For this review, take the finished solid that the model builds, in its own axes (mm). Round coordinates to 2 decimals unless told otherwise and drop trailing zeros. Order: outer loops, then holes, each group sorted by start corner. A loop starts at its lowest first (then second) coordinate and runs counter-clockwise, first axis right, second up. Notation, with made-up numbers: M 54.25,31.5 L 106.25,31.5 A8 ccw 106.25,41.5 Z; hole C 15,-26 d1. An arc over 180 degrees is marked long. Answer as a JSON object with one key per item and string values.
from build123d import *

# Parameters (mm, degrees)
F1_DEPTH = 250


# Not quite as in the source:
# - a fillet or chamfer that OpenCascade refuses, or shapes differently, is made with other operations: its cross-section is extruded or revolved along the edge and cut away or added


with BuildPart() as f1:
    # F0 (on Front) → F1 (new body)
    with BuildSketch(Plane.XZ):
        with BuildLine():
            ThreePointArc((14.3910080635, 0), (-13.3075418668, 5.4781787619), (10.2202866776, -10.1314783379))
            ThreePointArc((10.2202866776, -10.1314783379), (13.3075418668, -5.4781787619), (14.3910080635, 0))
        make_face()
        with BuildLine():
            ThreePointArc((8.400959745, -10.0958666852), (-11.8920367391, 5.5751332681), (13.1340263728, 0))
            ThreePointArc((13.1340263728, 0), (12.3705279138, -4.4127868626), (10.168798903, -8.3125313612))
            ThreePointArc((10.168798903, -8.3125313612), (10.4759385173, -8.7353566894), (10.5845781271, -9.2465449483))
            ThreePointArc((10.5845781271, -9.2465449483), (10.4899428261, -9.7250361614), (10.2202866776, -10.1314783379))
            ThreePointArc((10.2202866776, -10.1314783379), (9.3029968872, -10.5032859052), (8.400959745, -10.0958666852))
        make_face(mode=Mode.SUBTRACT)
        with BuildLine():
            ThreePointArc((10.168798903, -8.3125313612), (9.3275964364, -9.2465449483), (8.400959745, -10.0958666852))
            ThreePointArc((8.400959745, -10.0958666852), (9.3029968872, -10.5032859052), (10.2202866776, -10.1314783379))
            ThreePointArc((10.2202866776, -10.1314783379), (10.4899428261, -9.7250361614), (10.5845781271, -9.2465449483))
            ThreePointArc((10.5845781271, -9.2465449483), (10.4759385173, -8.7353566894), (10.168798903, -8.3125313612))
        make_face()
    extrude(amount=F1_DEPTH)

    # F2: fillet of radius 5 on 1 edges, made by hand

    # F2_s1 → F2_t2 (revolve, cut)
    with BuildSketch(Plane(origin=(0, 0, 0), x_dir=(0, 1, 0), z_dir=(-0.7040144994, 0, -0.7101855987))):
        with BuildLine():
            ThreePointArc((-246.6849111722, 14.3910080635), (-248.4576080518, 14.0662134893), (-250, 13.1340263728))
            Line((-250, 13.1340263728), (-250, 14.3910080635))
            Line((-250, 14.3910080635), (-246.6849111722, 14.3910080635))
        make_face()
    revolve(axis=Axis((0, -250, 0), (0, -1, 0)), mode=Mode.SUBTRACT)


solid = f1.part
1) Add section B-B on y = -172. State the section outline as (x, z) points.
Geometry check:
{"outline": "C 0,0 d28.78; hole C 0,0 d26.27"}
2) Insertion check: P1, Ø12, axis at y = -211, z = -4, coming from the +X side; P2, Ø8, axis at x = 6.5, y = -209.5, coming from the -Z side; P3, Ø3, axis at x = -11.5, y = -93.5, coming from the -Z side; P4, Ø2, axis at x = 2.5, y = -46.5, coming from the -Z side. Each pin has a flat end and moves straight along its axis. Give the tip position at first contact, or say it passes through.
Geometry check:
{"P1": "stops at x = 14.39", "P2": "stops at z = -14.17", "P3": "stops at z = -10.35", "P4": "stops at z = -14.31"}
3) For L1, parallel to Z at x = 0, y = -100.5; L2, parallel to X at y = -198, z = 6.25; L3, parallel to X at y = -236.5, z = 8.75, list the stretches that pass through material, from the lowest coordinate up.
Geometry check:
{"L1": "z = -14.39 to -13.13, 13.13 to 14.39", "L2": "x = -12.96 to -11.55, 11.55 to 12.96", "L3": "x = -11.43 to -9.79, 9.79 to 11.43"}
4) Add section A-A on x = 0. State the section outline as (y, z) points.
Geometry check:
{"outline": "M -250,-13.13 A5 ccw -246.68,-14.39 L 0,-14.39 L 0,-13.13 Z; M -250,13.13 L 0,13.13 L 0,14.39 L -246.68,14.39 A5 ccw Z"}
